Could you check a few things on this model? Use its own coordinates, in mm. Face numbers are marked on the shaded views. A direction names the side the tool comes from. Round coordinates to 2 decimals unless told otherwise and drop trailing zeros. Write each loop counter-clockwise with the first axis right and the second up, starting at its lowest first coordinate (ties: lowest second). Pieces come first, ordered by that corner, then holes. Notation, with made-up numbers: (-35.5, 86) -> (-13.5, 86) arc R19 cw to (-13.5, 100) -> close; hole circle Ø8 at (63, 71). An arc over 180 degrees is marked (long way). Answer in a Markdown table with one row per item.
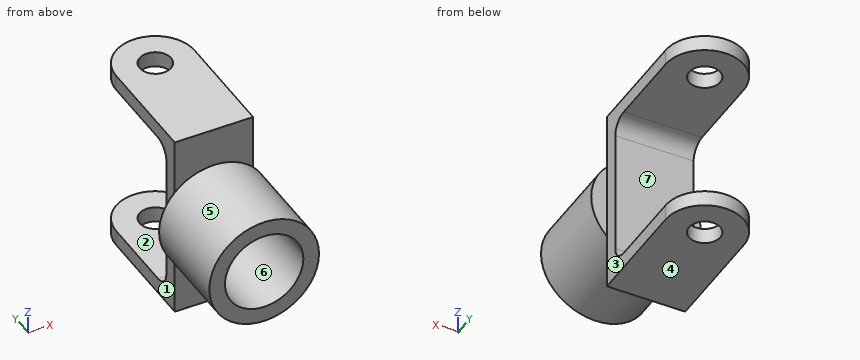
Autodesk Inventor part; units mm, degrees
ref_plane "YZ Plane" through (0, 0, 0) normal (1, 0, 0) x (0, 1, 0)
ref_plane "XZ Plane" through (0, 0, 0) normal (0, 1, 0) x (-1, 0, 0)
ref_plane "XY Plane" through (0, 0, 0) normal (0, 0, 1) x (1, 0, 0)
sketch "Sketch1" plane through (0, 0, 0) normal (0, 0, 1) x (1, 0, 0)
  circle A0 centre (0, 0) radius 5
  circle A1 centre (0, 0) radius 12.5
  line L0 (-12.5, 0) -> (12.5, 0)
  line L1 (12.5, 0) -> (12.5, -30)
  line L2 (12.5, -30) -> (-12.5, -30)
  line L3 (-12.5, -30) -> (-12.5, 0)
  dimension "d1" = 25
  dimension "d0" = 10
  dimension "d2" = 25
  dimension "d3" = 30
extrude "Extrusion1" add sketch "Sketch1" along normal blind 5 contours L0 A1 A0 | A0 L0 A1 | L1 L2 L3 A1
pattern_linear "Rectangular Pattern1" count 2 spacing 55 along (0, 0, 1) of "Extrusion1"
sketch "Sketch2" plane through (-12.5, -30, 55) normal (0, -1, 0) x (1, 0, 0)
  line L0 (0, 5) -> (25, 5)
  line L1 (25, 5) -> (0, 5)
  line L2 (0, 5) -> (0, -55)
  line L3 (0, -55) -> (25, -55)
  line L4 (25, -55) -> (25, 5)
  point P0 (12.5, -55)
extrude "Extrusion2" add sketch "Sketch2" along normal blind 5
fillet "Fillet1" radius 5 2 edges at (0, -30, 5) (0, -30, 55)
sketch "Sketch3" plane through (-12.5, -35, 55) normal (0, -1, 0) x (1, 0, 0)
  circle A0 centre (12.5, -25) radius 17.5
  circle A1 centre (12.5, -25) radius 12.5
  line L0 (0, -55) -> (25, -55)
  point P0 (12.5, -55)
  dimension "d12" = 35
  dimension "d15" = 30
extrude "Extrusion3" add sketch "Sketch3" along normal blind 30
properties part number "uJoint.1"
1) Imagine slicing it at D-D, the plane x = 9.5. Please give me the cut outline in (y, z), plus the area to 3 significant figures.
Findings:
| item | result |
|---|---|
| outline | (-65, 15.3) -> (-35, 15.3) -> (-35, 0) -> (8.12, 0) -> (8.12, 5) -> (-25, 5) arc R5 cw to (-30, 10) -> (-30, 50) arc R5 cw to (-25, 55) -> (8.12, 55) -> (8.12, 60) -> (-35, 60) -> (-35, 44.7) -> (-65, 44.7) -> (-65, 38.12) -> (-35, 38.12) -> (-35, 21.88) -> (-65, 21.88) -> close |
| area | 1,090 mm^2 |
2) Please list where these lines run through material, in increasing order: line 1 (X direction, y = 0, z = 56.1); line 2 (Z direction, x = 9.5, y = -14.5); line 3 (Y direction, x = 0, z = 3).
Findings:
| item | result |
|---|---|
| line 1 | x = -12.5 to -5, 5 to 12.5 |
| line 2 | z = 0 to 5, 55 to 60 |
| line 3 | y = -35 to -5, 5 to 12.5 |
3) Imagine slicing it at C-C, the plane z = 23. Please give me the cut outline in (x, y), plus the area to 3 significant figures.
Findings:
| item | result |
|---|---|
| outline | (-16.04, -65) -> (-10.36, -65) -> (-10.36, -35) -> (10.36, -35) -> (10.36, -65) -> (16.04, -65) -> (16.04, -35) -> (12.5, -35) -> (12.5, -30) -> (-12.5, -30) -> (-12.5, -35) -> (-16.04, -35) -> close |
| area | 466 mm^2 |
4) Imagine slicing it at B-B, the plane x = 2. Please give me the cut outline in (y, z), plus the area to 3 significant figures.
Findings:
| item | result |
|---|---|
| outline | (-65, 12.61) -> (-35, 12.61) -> (-35, 0) -> (-4.58, 0) -> (-4.58, 5) -> (-25, 5) arc R5 cw to (-30, 10) -> (-30, 50) arc R5 cw to (-25, 55) -> (-4.58, 55) -> (-4.58, 60) -> (-35, 60) -> (-35, 47.39) -> (-65, 47.39) -> (-65, 42.34) -> (-35, 42.34) -> (-35, 17.66) -> (-65, 17.66) -> close; (4.58, 0) -> (12.34, 0) -> (12.34, 5) -> (4.58, 5) -> close; (4.58, 55) -> (12.34, 55) -> (12.34, 60) -> (4.58, 60) -> close |
| area | 945 mm^2 |
5) Imagine slicing it at A-A, the plane y = -23. Please give me the cut outline in (x, z), plus the area to 3 significant figures.
Findings:
| item | result |
|---|---|
| outline | (-12.5, 0) -> (12.5, 0) -> (12.5, 5) -> (-12.5, 5) -> close; (-12.5, 55) -> (12.5, 55) -> (12.5, 60) -> (-12.5, 60) -> close |
| area | 250 mm^2 |
6) For the marked faces 1, 2 and 3, which set-ups out of +Z, -Z, +X, -X, +Y, -Y let a thin tool reach every point of the face, with its end or its side?
Findings:
| item | result |
|---|---|
| face 1 | +Z, -Z, -X, +Y |
| face 2 | +X, -X, +Y |
| face 3 | +Z, -Z, +X, +Y |
7) For pin 1 (8 mm diameter, centred on x = 10.5, z = 33, fed in from +Y); pin 2 (4 mm diameter, centred on x = 15, z = 30, fed in from +Y); pin 3 (12 mm diameter, centred on x = 4, z = 35.5, fed in from -Y); pin 4 (4 mm diameter, centred on y = -48.5, z = 23.5, fed in from -X), each with a flat end and sliding along its axis, tell me the tip position at first contact or that it passes through.
Findings:
| item | result |
|---|---|
| pin 1 | stops at y = -30 |
| pin 2 | stops at y = -35 |
| pin 3 | stops at y = -65 |
| pin 4 | stops at x = -16.91 |
8) Thinking about a two-plate mould opening in Z: for the marked faces 4, 5, 6 and 7, which applies, +Z half, -Z half, draft (parallel to the pull), parting line (faces both ways), or undercut?
Findings:
| item | result |
|---|---|
| face 4 | -Z half |
| face 5 | parting line |
| face 6 | undercut |
| face 7 | undercut |
